```python
from build123d import *

# Parameters (mm, degrees)
F0_W     = 30.48
F0_H     = 31.75
F0_R     = 3.4925
F1_DEPTH = 6.35
F2_W     = 30.48
F2_H     = 31.75
F3_DEPTH = 12.7
F4_W     = 11.1125
F4_H     = 30.1625
F5_DEPTH = 1.5875
F6_W     = 11.43
F6_H     = 30.1625
F7_DEPTH = 1.5875
F8_R     = 2.38125
F9_DEPTH = 28.8935


with BuildPart() as f1:
    # F0 (on Front) → F1 (new body)
    with BuildSketch(Plane.XZ):
        with Locations((-15.24, 15.875)):
            Rectangle(F0_W, F0_H)
        with Locations((-24.13, 6.35)):
            Circle(F0_R, mode=Mode.SUBTRACT)
        with Locations((-24.13, 15.24)):
            Circle(F0_R, mode=Mode.SUBTRACT)
        with Locations((-15.24, 6.35)):
            Circle(F0_R, mode=Mode.SUBTRACT)
        with Locations((-6.35, 6.35)):
            Circle(F0_R, mode=Mode.SUBTRACT)
        with Locations((-15.24, 15.24)):
            Circle(F0_R, mode=Mode.SUBTRACT)
        with Locations((-6.35, 15.24)):
            Circle(F0_R, mode=Mode.SUBTRACT)
        with Locations((-24.13, 24.13)):
            Circle(F0_R, mode=Mode.SUBTRACT)
        with Locations((-15.24, 24.13)):
            Circle(F0_R, mode=Mode.SUBTRACT)
        with Locations((-6.35, 24.13)):
            Circle(F0_R, mode=Mode.SUBTRACT)
    extrude(amount=F1_DEPTH)

    # F2 (on face) → F3 (join)
    with BuildSketch(Plane(origin=(0, 0, 0), x_dir=(-1, 0, 0), z_dir=(0, 1, 0))):
        with Locations((15.24, 15.875)):
            Rectangle(F2_W, F2_H)
    extrude(amount=F3_DEPTH)

    # F4 (on face) → F5 (cut)
    with BuildSketch(Plane.YZ):
        with Locations((4.98475, 15.08125)):
            Rectangle(F4_W, F4_H)
    extrude(amount=-F5_DEPTH, mode=Mode.SUBTRACT)

    # F6 (on face) → F7 (cut)
    with BuildSketch(Plane(origin=(-30.48, 0, 0), x_dir=(0, -1, 0), z_dir=(-1, 0, 0))):
        with Locations((-4.826, 15.08125)):
            Rectangle(F6_W, F6_H)
    extrude(amount=-F7_DEPTH, mode=Mode.SUBTRACT)

    # F8 (on face) → F9 (cut, through all)
    with BuildSketch(Plane(origin=(-28.8925, 0, 0), x_dir=(0, -1, 0), z_dir=(-1, 0, 0))):
        with Locations((-4.826, 23.8125)):
            Circle(F8_R)
        with Locations((-4.826, 7.9375)):
            Circle(F8_R)
    extrude(amount=-F9_DEPTH, mode=Mode.SUBTRACT)


solid = f1.part
```
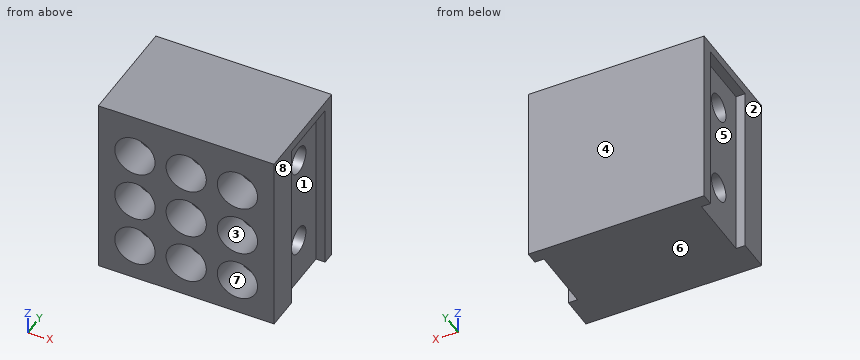
Can you work these out from the model? Positions are in its coordinate system, mm. Face numbers are marked on the shaded views. A direction names the side the tool comes from. Coordinates: 2 decimals unless noted, no trailing zeros. Loops run counter-clockwise (first coordinate to the right, second up) from the corner with the lowest first, then second, coordinate; pieces in that order, holes last. Notation, with made-up numbers: (-2, 79.25) - (6, 79.25) arc R21 ccw to (6, 108.25) - close; hole circle Ø4 at (43.25, 89). An arc over 180 degrees is marked (long way). Answer as CSV lines item,"result". Start each with the question number.
1) Which directions (+Z, -Z, +X, -X, +Y, -Y) give clear straight access to the entire face, cutting with the end or side of a thin tool? Please do the marked faces 1, 2, 3, 4 and 5.
2) Suppose I cut it at A-A (y = 1). Please give me the cut outline in (x, z), plus the area to 3 significant figures.
3) For pin 1 (3.5 mm diameter, centred on x = -6, z = 15, fed in from -Y); pin 2 (3.5 mm diameter, centred on y = 2, z = 20.5, fed in from +X); pin 3 (4 mm diameter, centred on y = 4.83, z = 7.94, fed in from +X); pin 4 (0.5 mm diameter, centred on x = -29.5, y = 4, fed in from -Z), each with a flat end and sliding along its axis, tell me the tip position at first contact or that it passes through.
4) I need wall thicknesses on line 1 (Z direction, x = -24.13, y = -4); line 2 (Z direction, x = -22.5, y = -2); line 3 (Z direction, x = -3.5, y = 3.25). Which ranges of each line are inside material? Lowest first, please. Write a range as from..to.
5) Suppose I cut it at D-D (z = 15.24). Please give me the cut outline in (x, y), plus the area to 3 significant figures.
6) Thinking about a two-plate mould opening in Z: for the marked faces 6, 7 and 8, which applies, pulls with the +Z half, pulls with the -Z half, needs draft (parallel to the pull), parting line crosses it, or undercut?
7) Suppose I cut it at C-C (x = -6.35). Please give me the cut outline in (y, z), plus the area to 3 significant figures.
8) Suppose I cut it at B-B (z = 7). Please give me the cut outline in (x, y), plus the area to 3 significant figures.
Check result:
1,face 1,"-Z, +X"
1,face 2,"+Z, -Z, -X, +Y, -Y"
1,face 3,"-Y"
1,face 4,"+Z, -Z, +X, -X, +Y"
1,face 5,"-Z, -X"
2,outline,"(-30.48, 30.16) - (-28.89, 30.16) - (-28.89, 0) - (-1.59, 0) - (-1.59, 30.16) - (0, 30.16) - (0, 31.75) - (-30.48, 31.75) - close"
2,area,"872 mm²"
3,pin 1,"stops at y = 0"
3,pin 2,"stops at x = -1.59"
3,pin 3,"passes through"
3,pin 4,"stops at z = 30.16"
4,line 1,"z = 0..2.86, 9.84..11.75, 18.73..20.64, 27.62..31.75"
4,line 2,"z = 0..3.26, 9.44..12.15, 18.33..21.04, 27.22..31.75"
4,line 3,"z = 0..6.15, 9.72..22.03, 25.6..31.75"
5,outline,"(-30.48, -6.35) - (-27.62, -6.35) - (-27.62, 0) - (-20.64, 0) - (-20.64, -6.35) - (-18.73, -6.35) - (-18.73, 0) - (-11.75, 0) - (-11.75, -6.35) - (-9.84, -6.35) - (-9.84, 0) - (-2.86, 0) - (-2.86, -6.35) - (0, -6.35) - (0, -0.57) - (-1.59, -0.57) - (-1.59, 10.54) - (0, 10.54) - (0, 12.7) - (-30.48, 12.7) - (-30.48, 10.54) - (-28.89, 10.54) - (-28.89, -0.89) - (-30.48, -0.89) - close"
5,area,"412 mm²"
6,face 6,"pulls with the -Z half"
6,face 7,"undercut"
6,face 8,"needs draft"
7,outline,"(-6.35, 0) - (12.7, 0) - (12.7, 31.75) - (-6.35, 31.75) - (-6.35, 27.62) - (0, 27.62) - (0, 20.64) - (-6.35, 20.64) - (-6.35, 18.73) - (0, 18.73) - (0, 11.75) - (-6.35, 11.75) - (-6.35, 9.84) - (0, 9.84) - (0, 2.86) - (-6.35, 2.86) - close; hole circle Ø4.76 at (4.83, 7.94); hole circle Ø4.76 at (4.83, 23.81)"
7,area,"436 mm²"
8,outline,"(-30.48, -6.35) - (-27.56, -6.35) - (-27.56, 0) - (-20.7, 0) - (-20.7, -6.35) - (-18.67, -6.35) - (-18.67, 0) - (-11.81, 0) - (-11.81, -6.35) - (-9.78, -6.35) - (-9.78, 0) - (-2.92, 0) - (-2.92, -6.35) - (0, -6.35) - (0, -0.57) - (-1.59, -0.57) - (-1.59, 2.64) - (-28.89, 2.64) - (-28.89, -0.89) - (-30.48, -0.89) - close; (-30.48, 10.54) - (-28.89, 10.54) - (-28.89, 7.01) - (-1.59, 7.01) - (-1.59, 10.54) - (0, 10.54) - (0, 12.7) - (-30.48, 12.7) - close"
8,area,"295 mm²"
